from build123d import *

# Parameters (mm, degrees)
SKETCH_1_R      = 5.5
SKETCH_1_R_2    = 2
EXTRUDE_1_DEPTH = 1
SKETCH_2_R      = 2
EXTRUDE_2_DEPTH = 4.5


with BuildPart() as part:
    # 草图1 → 凸台-拉伸1 (new body)
    with BuildSketch(Plane(origin=(0, 0, 0), x_dir=(1, 0, 0), z_dir=(0, 1, 0))):
        with Locations(Location((0, 0, 0), (0, 0, 270))):
            Circle(SKETCH_1_R)
        with Locations(Location((0, 0, 0), (0, 0, 270))):
            Circle(SKETCH_1_R_2, mode=Mode.SUBTRACT)
    extrude(amount=EXTRUDE_1_DEPTH)

    # 草图2 → 凸台-拉伸2 (add)
    with BuildSketch(Plane(origin=(0, 1, 0), x_dir=(1, 0, 0), z_dir=(0, 1, 0))):
        Polygon((4.618802154, 0), (2.309401077, 4), (-2.309401077, 4), (-4.618802154, 0), (-2.309401077, -4), (2.309401077, -4), align=None)
        with Locations(Location((0, 0, 0), (0, 0, 270))):
            Circle(SKETCH_2_R, mode=Mode.SUBTRACT)
    extrude(amount=EXTRUDE_2_DEPTH)

    # 草图3 → 切除-旋转1 (revolve, cut)
    with BuildSketch(Plane.XY):
        with BuildLine():
            ThreePointArc((-3.2, 5.5), (-3.686821507, 5.219718819), (-3.9, 4.7))
            Line((-3.9, 4.7), (-4, 4.7))
            ThreePointArc((-4, 4.7), (-4.441923124, 4.467149897), (-4.618802154, 4))
            Line((-4.618802154, 4), (-4.618802154, 5.5))
            Line((-4.618802154, 5.5), (-3.2, 5.5))
        make_face()
    revolve(axis=Axis((0, 5.5, 0), (0, -1, 0)), mode=Mode.SUBTRACT)


solid = part.part
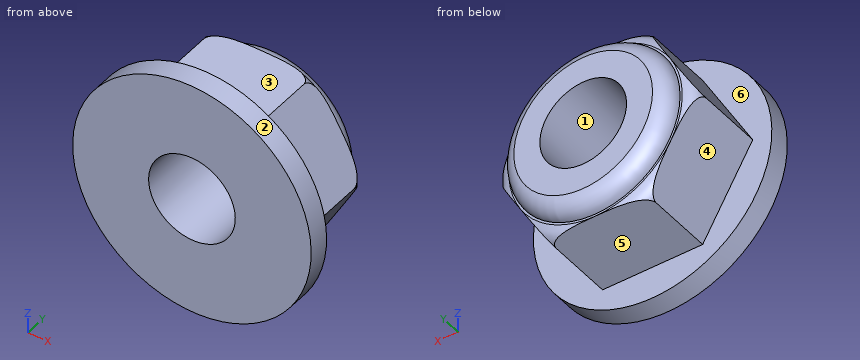
CAD build for the part. Positions are in the model's coordinates, mm. Face numbers are marked on the shaded views. A direction names the side the tool comes from. Round coordinates to 2 decimals unless told otherwise and drop trailing zeros. Loops run counter-clockwise (first coordinate to the right, second up) from the corner with the lowest first, then second, coordinate; pieces in that order, holes last.
(1) Cut at A-A (y = 1.45). Give the cut face in (x, z).
(2) Cut at B-B (z = -4.5). Give the cut face in (x, y).
(3) Cut at C-C (y = 4.85). Give the cut face in (x, z).
(4) Drop flat-ended pins along their axis: pin 1 (1.1 mm diameter, centred on x = -1, y = 2.5, fed in from +Z); pin 2 (1.9 mm diameter, centred on x = -1, y = 3.5, fed in from -Z); pin 3 (2 mm diameter, centred on x = 1.5, z = 4, fed in from +Y). Give the stop position or say it passes through.
(5) Which spindle directions (+Z, -Z, +X, -X, +Y, -Y) get a long thin tool onto all of the face, cutting with end or side? Do the marked faces 4, 5 and 6. Say none if no direction does.
(6) Wall check: line 1 along Y through (x, z) = (-1, 4.25); line 2 along Z through (x, y) = (-0.5, 5.3); line 3 along Z through (x, y) = (0.25, 1.4). Give the ranges that are in metal, low to high.
(7) Two-plate mould, pull along Z, no slides. Class the marked faces 1, 2 and 3: +Z half, -Z half, draft (parallel to the pull), parting line (faces both ways), or undercut.
Findings below:
1. outline: (-4.62, 0) - (-2.31, -4) - (2.31, -4) - (4.62, 0) - (2.31, 4) - (-2.31, 4) - close; hole circle Ø4 at (0, 0)
2. outline: (-3.16, 0) - (3.16, 0) - (3.16, 1) - (-3.16, 1) - close
3. outline: circle Ø7.76 at (0, 0); hole circle Ø4 at (0, 0)
4. pin 1: stops at z = 4
4. pin 2: stops at z = -4
4. pin 3: stops at y = 5.48
5. face 4: -Z, -X, +Y
5. face 5: -Z, +X, -X, +Y
5. face 6: +Y
6. line 1: y = 0 to 1
6. line 2: z = -3.57 to -1.94, 1.94 to 3.57
6. line 3: z = -4 to -1.98, 1.98 to 4
7. face 1: undercut
7. face 2: parting line
7. face 3: +Z half
